Geometry check sheet. Reference: drawing and pictorial views, mm from the part's lowest x, y, z. Coordinates: 2 decimals unless noted, no trailing zeros. Write each loop counter-clockwise with the first axis right and the second up, starting at its lowest first coordinate (ties: lowest second). Pieces come first, ordered by that corner, then holes. Notation, with made-up numbers: (77.25, 53.25) -> (100.25, 53.25) arc R20 ccw to (100.25, 61.25) -> close; hole circle Ø8 at (4, 58). An arc over 180 degrees is marked (long way). Use a Markdown table: item, result. Add a question column.
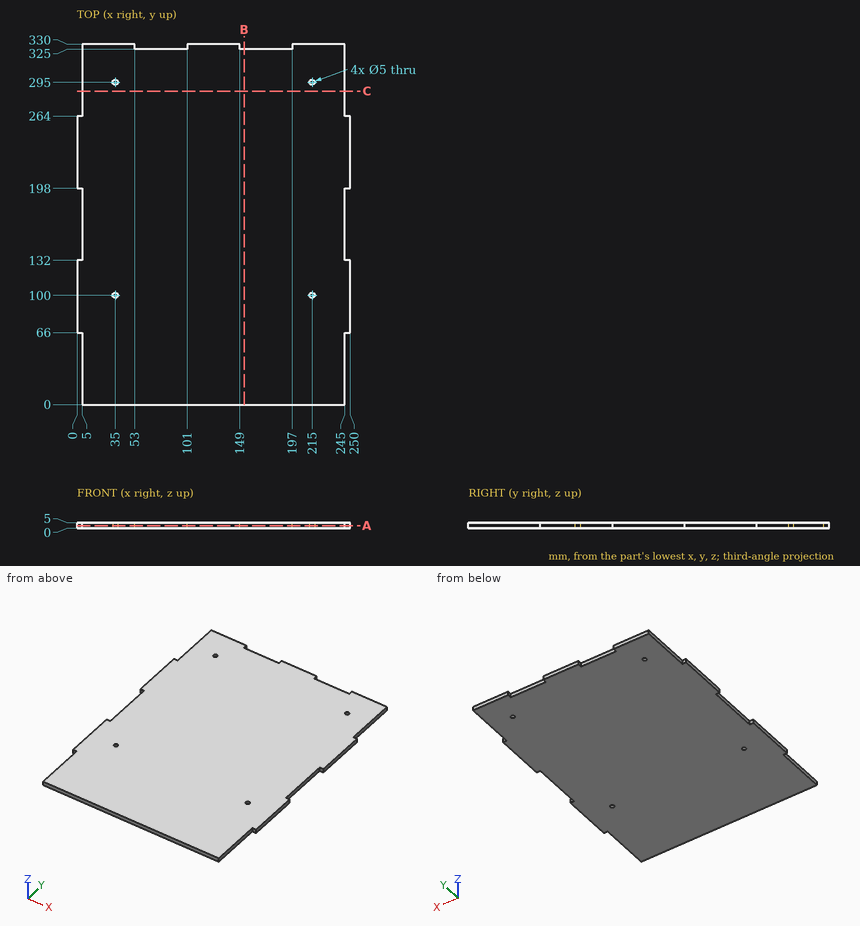
1) Cross-section at B-B on x = 153. Record the boundary of the cut face in (y, z), then the cut area to 4 significant figures.
2) Thickness scan on L1, parallel to Y at x = 215, z = 3.9; L2, parallel to Y at x = 166.5, z = 3.9; L3, parallel to X at y = 158, z = 4. Record the ranges inside material, lowest first.
3) Cross-section at C-C on y = 287. Record the boundary of the cut face in (x, z).
4) Gauge pin test, flat ends, axial feed: pin 1 (1.5 mm diameter, centred on x = 247, z = 1.5, fed in from +Y); pin 2 (6.5 mm diameter, centred on x = 35, y = 100, fed in from -Z); pin 3 (2.5 mm diameter, centred on x = 248.5, z = 1.5, fed in from -Y); pin 4 (2 mm diameter, centred on x = 63.5, z = 3.5, fed in from +Y). Record the tip position at first contact, or that the pin passes through.
5) Cross-section at A-A on z = 2.45. Give the number of separate pieces and of enclosed holes in the cut face, then the cut area to 3 significant figures.
Returned:
| question | item | result |
|---|---|---|
| 1 | outline | (0, 0) -> (325, 0) -> (325, 5) -> (0, 5) -> close |
| 1 | area | 1,625 mm² |
| 2 | L1 | y = 0 to 97.5, 102.5 to 292.5, 297.5 to 330 |
| 2 | L2 | y = 0 to 325 |
| 2 | L3 | x = 5 to 245 |
| 3 | outline | (5, 0) -> (245, 0) -> (245, 5) -> (5, 5) -> close |
| 4 | pin 1 | stops at y = 264 |
| 4 | pin 2 | stops at z = 0 |
| 4 | pin 3 | stops at y = 66 |
| 4 | pin 4 | stops at y = 325 |
| 5 | separate pieces | 1 |
| 5 | enclosed holes | 4 |
| 5 | area | 80,000 mm² |
